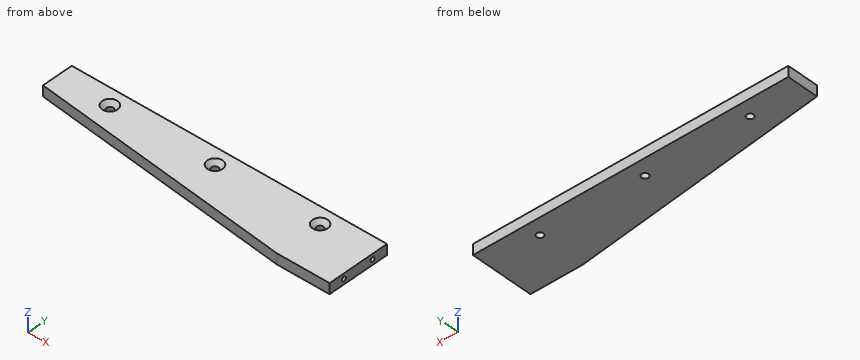
Autodesk Inventor part; units mm, degrees
ref_plane "YZ Plane" through (0, 0, 0) normal (1, 0, 0) x (0, 1, 0)
ref_plane "XZ Plane" through (0, 0, 0) normal (0, 1, 0) x (-1, 0, 0)
ref_plane "XY Plane" through (0, 0, 0) normal (0, 0, 1) x (1, 0, 0)
sketch "Esboço1" plane through (0, 0, 0) normal (0, 0, 1) x (1, 0, 0)
  line L0 (-210, 0) -> (210, 0) construction
  line L1 (0, -42) -> (0, 42) construction
  line L2 (-150, 30) -> (150, 30)
  line L3 (150, 30) -> (150, -30)
  line L4 (150, -30) -> (-150, -30)
  line L5 (-150, -30) -> (-150, 30)
  line L6 (-150, 15) -> (150, 15) construction
  line L7 (-150, -15) -> (150, -15) construction
  line L8 (-150, 0) -> (100, -30)
  point P0 (0, 0)
  point P1 (-100, 15)
  point P2 (-100, -15)
  point P3 (100, 15)
  point P4 (100, -15)
  point P5 (0, 15)
  point P6 (0, -15)
  dimension "d0" = 60
  dimension "d1" = 300
  dimension "d2" = 30
  dimension "d3" = 100
  dimension "d24" = 250
extrude "Extrusão1" add sketch "Esboço1" along normal mid plane 10 contours L2 L3 L4 L8 L5
sketch "Esboço2" plane through (0, 0, 5) normal (0, 0, 1) x (1, 0, 0)
  point P0 (0, 0)
  point P1 (-100, 15)
  point P2 (-100, -15)
  point P3 (0, 15)
  point P4 (0, -15)
  point P5 (100, 15)
  point P6 (100, -15)
hole "Furo1" at (-100, 15, 5) at (0, 15, 5) at (100, 15, 5) direction (0, 0, -1) diameter 6.5 end through all countersink diameter 14.5 countersink angle 90
sketch "Esboço3" plane through (150, -30, 5) normal (1, 0, 0) x (0, 0, -1)
  line L0 (12, 30) -> (-2, 30) construction
  line L1 (5, -12) -> (5, 72) construction
  point P0 (5, 30)
  point P1 (5, 45)
  point P2 (5, 15)
  dimension "d16" = 30
hole "Furo2" at (150, 15, 0) at (150, -15, 0) direction (-1, 0, 0) diameter 4.134 depth 20 tip angle 118
properties part number "Chapa Suporte 2R (Trilho Roletado)" material "Aluminio 1060"
Input: part model. Units: mm. Frame: model coordinates. Coordinates: 2 decimals unless noted, no trailing zeros. Order: outer loops, then holes, each group sorted by start corner. A loop starts at its lowest first (then second) coordinate and runs counter-clockwise, first axis right, second up. Notation, with made-up numbers: M 78.25,81.5 L 137.25,81.5 A26 cw 137.25,108.5 Z; hole C -14.5,23 d9. An arc over 180 degrees is marked long. Write item = value, one per line. Start each with the question number.
(1) Section B-B on x = 0. Output: boundary loops of the cut face in (y, z).
(2) Section C-C on x = -34.5. Output: boundary loops of the cut face in (y, z).
(3) Section A-A on x = -100. Output: boundary loops of the cut face in (y, z), and give its area (3 significant figures).
(4) Line query: line 1 along X through (y, z) = (15, -3.8); line 2 along Y through (x, z) = (134, 0); line 3 along Z through (x, y) = (140, -15). Output: solid intervals per line, ascending. Write a range as [from, to].
(5) First-contact query: P1, Ø8.5, axis at x = -100, y = 15, coming from the +Z side; P2, Ø3.5, axis at y = 15, z = 0, coming from the +X side; P3, Ø2.5, axis at y = -15, z = 0, coming from the +X side; P4, Ø5, axis at x = 100, y = 15, coming from the -Z side. Flat tips, straight axial feed; report the tip coordinate or a pass-through.
Result set:
q1.outline = M -18,-5 L 11.75,-5 L 11.75,1 L 7.75,5 L -18,5 Z; M 18.25,-5 L 30,-5 L 30,5 L 22.25,5 L 18.25,1 Z
q2.outline = M -13.86,-5 L 30,-5 L 30,5 L -13.86,5 Z
q3.outline = M -6,-5 L 11.75,-5 L 11.75,1 L 7.75,5 L -6,5 Z; M 18.25,-5 L 30,-5 L 30,5 L 22.25,5 L 18.25,1 Z
q3.area = 279 mm²
q4.line_1 = [-150, -103.25], [-96.75, -3.25], [3.25, 96.75], [103.25, 150]
q4.line_2 = [-30, -17.07], [-12.93, 12.93], [17.07, 30]
q4.line_3 = [-5, -2.07], [2.07, 5]
q5.P1 = 2
q5.P2 = 129.81
q5.P3 = 129.51
q5.P4 = through
